from build123d import *

# Parameters (mm, degrees)
F0_R      = 11
F1_DEPTH  = 3
F2_R      = 5.75
F3_DEPTH  = 1.2
F4_R      = 2.5
F5_DEPTH  = 7
F6_R      = 0.6
F10_DEPTH = 7
F11_W     = 1.2
F11_H     = 2.8315826069
F11_H_2   = 1.2
F11_W_2   = 2.9928033758
F12_DEPTH = 4
F13_R     = 0.4
F14_R     = 1
F15_R     = 0.2


# Not quite as in the source:
# - a feature of the source that left no trace in its solid (it failed there, or was rolled back) is left out


with BuildPart() as f1:
    # F0 (on Top) → F1 (new body)
    with BuildSketch(Plane.XY):
        Circle(F0_R)
    extrude(amount=F1_DEPTH)

    # F2 (on face) → F3 (join)
    with BuildSketch(Plane.XY.offset(3)):
        Circle(F2_R)
    extrude(amount=F3_DEPTH)

    # F4 (on face) → F5 (join)
    with BuildSketch(Plane.XY.offset(4.2)):
        Circle(F4_R)
    extrude(amount=F5_DEPTH)

    # F6 (on face) → F10 (cut)
    with BuildSketch(Plane.XY.offset(11.2)):
        Circle(F6_R)
    extrude(amount=-F10_DEPTH, mode=Mode.SUBTRACT)

    # F11 (on face) → F12 (cut)
    with BuildSketch(Plane.XY.offset(11.2)):
        with Locations((0, 2.0157913034)):
            Rectangle(F11_W, F11_H)
        Rectangle(F11_W, F11_H_2)
        with Locations((-2.0964016879, 0)):
            Rectangle(F11_W_2, F11_H_2)
        with Locations((2.0964016879, 0)):
            Rectangle(F11_W_2, F11_H_2)
        with Locations((0, -2.0157913034)):
            Rectangle(F11_W, F11_H)
    extrude(amount=-F12_DEPTH, mode=Mode.SUBTRACT)

    # F13
    f13_edges = [f1.edges().sort_by_distance(p)[0] for p in [
        (1.767767, -1.767767, 11.2),
        (-1.767767, -1.767767, 11.2),
        (-1.767767, 1.767767, 11.2),
        (1.767767, 1.767767, 11.2),
    ]]
    fillet(f13_edges, radius=F13_R)

    # F14
    f14_edges = [f1.edges().sort_by_distance(p)[0] for p in [
        (-11, 0, 3),
        (-11, 0, 0),
    ]]
    fillet(f14_edges, radius=F14_R)

    # F15
    f15_edges = [f1.edges().sort_by_distance(p)[0] for p in [
        (-0.6, 1.306231, 11.2),
        (-1.484924, 1.484924, 11.2),
        (-1.306231, 0.6, 11.2),
        (1.306231, 0.6, 11.2),
        (1.484924, 1.484924, 11.2),
        (0.6, 1.306231, 11.2),
        (0.6, -1.306231, 11.2),
        (1.484924, -1.484924, 11.2),
        (1.306231, -0.6, 11.2),
        (-1.306231, -0.6, 11.2),
        (-1.484924, -1.484924, 11.2),
        (-0.6, -1.306231, 11.2),
        (-0.6, 0, 7.2),
        (2.426932, -0.6, 9),
        (0.6, -2.426932, 9),
        (-0.6, -2.426932, 9),
        (-2.426932, -0.6, 9),
        (2.426932, 0.6, 9),
        (-2.426932, 0.6, 9),
        (0.6, 2.426932, 9),
        (-0.6, 2.426932, 9),
        (2.305572, -0.6, 11.08332),
        (0.6, -2.305572, 11.08332),
        (-0.6, -2.305572, 11.08332),
        (-2.305572, -0.6, 11.08332),
        (2.305572, 0.6, 11.08332),
        (0.6, 2.305572, 11.08332),
        (-2.305572, 0.6, 11.08332),
        (-0.6, 2.305572, 11.08332),
    ]]
    fillet(f15_edges, radius=F15_R)


solid = f1.part
Can you work these out from the model? Positions are in its coordinate system, mm. A direction names the side the tool comes from. Coordinates: 2 decimals unless noted, no trailing zeros. Write each loop counter-clockwise with the first axis right and the second up, starting at its lowest first coordinate (ties: lowest second). Pieces come first, ordered by that corner, then holes.
Q1. For P1, Ø0.8, axis at y = 1, z = 9.5, coming from the +X side; P2, Ø4, axis at x = -1, y = -6, coming from the -Z side; P3, Ø0.5, axis at y = -1.5, z = 9.5, coming from the +X side; P4, Ø5, axis at x = 4.5, z = 7.5, coming from the +Y side, each with a flat end and sliding along its axis, tell me the tip position at first contact or that it passes through.
Results found:
P1: stops at x = 2.36
P2: stops at z = 0
P3: stops at x = 2.17
P4: stops at y = 1.5
Q2. Imagine slicing it at B-B, the plane x = 0. List the corners of the cut face in (y, z) for me, plus the area to 3 significant figures.
Results found:
outline: (-11, 1) arc R1 ccw to (-10, 0) - (10, 0) arc R1 ccw to (11, 1) - (11, 2) arc R1 ccw to (10, 3) - (5.75, 3) - (5.75, 4.2) - (2.5, 4.2) - (2.5, 7.2) - (0.8, 7.2) arc R0.2 ccw to (0.6, 7) - (0.6, 4.2) - (-0.6, 4.2) - (-0.6, 7) arc R0.2 ccw to (-0.8, 7.2) - (-2.5, 7.2) - (-2.5, 4.2) - (-5.75, 4.2) - (-5.75, 3) - (-10, 3) arc R1 ccw to (-11, 2) - close
area: 90.3 mm2
Q3. Which directions (+Z, -Z, +X, -X, +Y, -Y) give clear straight access to the entire face, cutting with the end or side of a thin tool? Please do faces 4 (the face through (-1, -0.6, 9)), 5 (the face through (-0.6, 1, 9)), 6 (the face through (-0.75, 5.7, 3.59)), 7 (the face through (-1, 1, 11.2)), 8 (the face through (0, 0, 0)).
Results found:
face 4: +Z, +X, -X
face 5: +Z, +Y, -Y
face 6: +Z
face 7: +Z, +X, -X, +Y, -Y
face 8: -Z, +X, -X, +Y, -Y
Q4. Imagine slicing it at A-A, the plane z = 9. List the corners of the cut face in (x, y) for me, plus the area to 3 significant figures.
Results found:
outline: (-2.34, -0.87) arc R2.5 ccw to (-0.87, -2.34) arc R0.2 ccw to (-0.6, -2.16) - (-0.6, -0.6) - (-2.16, -0.6) arc R0.2 ccw to start; (-2.34, 0.87) arc R0.2 ccw to (-2.16, 0.6) - (-0.6, 0.6) - (-0.6, 2.16) arc R0.2 ccw to (-0.87, 2.34) arc R2.5 ccw to start; (0.6, -2.16) arc R0.2 ccw to (0.87, -2.34) arc R2.5 ccw to (2.34, -0.87) arc R0.2 ccw to (2.16, -0.6) - (0.6, -0.6) - close; (0.6, 0.6) - (2.16, 0.6) arc R0.2 ccw to (2.34, 0.87) arc R2.5 ccw to (0.87, 2.34) arc R0.2 ccw to (0.6, 2.16) - close
area: 9.05 mm2
Q5. If we mould it in two halves opening along X, with no side actions, what happens to faces 1 (the face through (0.6, -1, 9)), 2 (the face through (1.15, -2.22, 6.72)), 3 (the face through (1, 0.6, 9))? For each: +X half, -X half, draft (parallel to the pull), parting line (faces both ways), or undercut.
Results found:
face 1: undercut
face 2: parting line
face 3: draft
Q6. Please list where these lines run through material, in increasing order: L1, parallel to Y at x = 0, z = 5.05; L2, parallel to Z at x = -8, y = 1; L3, parallel to Z at x = -1, y = 5.5.
Results found:
L1: y = -2.5 to -0.6, 0.6 to 2.5
L2: z = 0 to 3
L3: z = 0 to 4.2
Q7. Imagine slicing it at D-D, the plane z = 3.5. List the corners of the cut face in (x, y) for me.
Results found:
outline: circle Ø11.5 at (0, 0)
